Could you check a few things on this drawing? It's one solid part, dimensions in mm from its lowest x, y, z. Round coordinates to 2 decimals unless told otherwise and drop trailing zeros. Loops run counter-clockwise (first coordinate to the right, second up) from the corner with the lowest first, then second, coordinate; pieces in that order, holes last. Notation, with made-up numbers: (-37.75, -1.5) -> (-29.75, -1.5) arc R27 cw to (-29.75, 29.5) -> close; hole circle Ø8 at (8.25, 26.25). An arc over 180 degrees is marked (long way). Write each question's results on one line, items separated by ' | '.
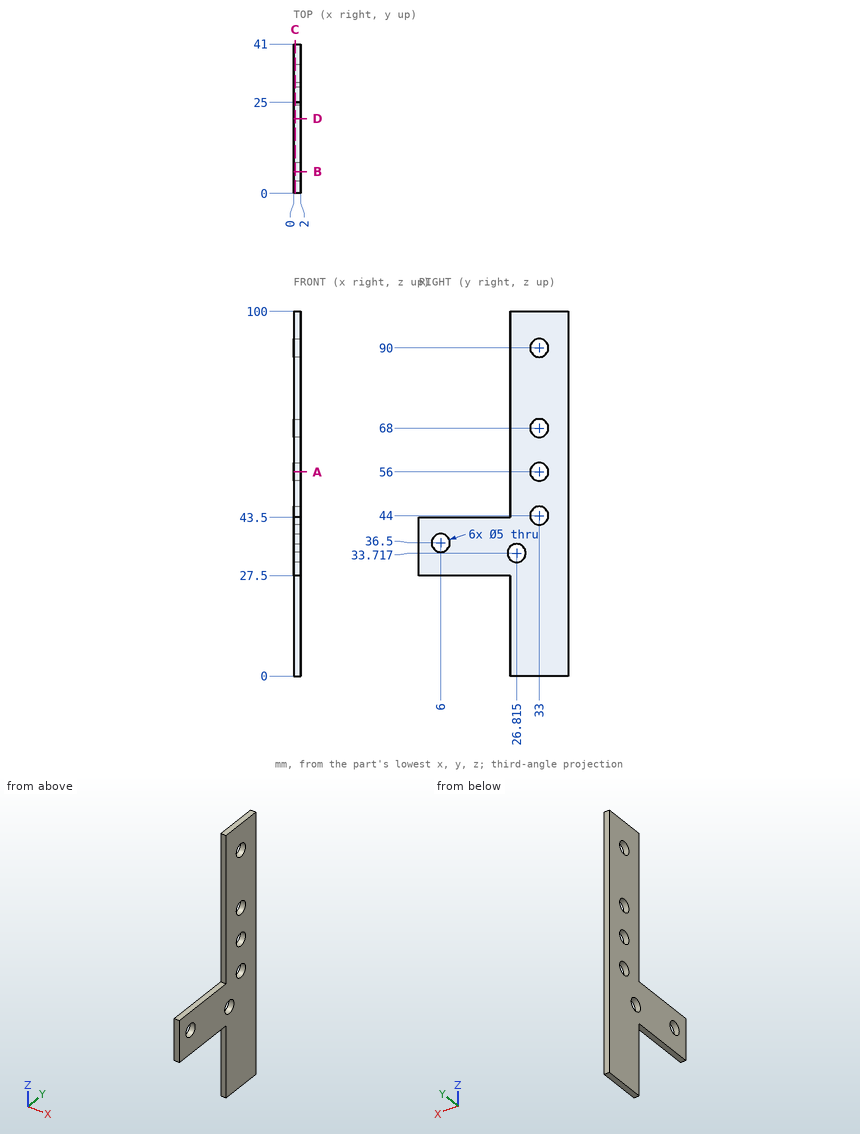
1) I'm going to push flat-ended pins straight in: pin 1 (4.5 mm diameter, centred on y = 26.81, z = 33.72, fed in from -X); pin 2 (0.6 mm diameter, centred on x = 1.5, z = 9, fed in from -Y). Where does each tip first touch, or does it pass through?
Model answer:
pin 1: passes through | pin 2: stops at y = 25
2) I want a section at B-B, the plane y = 6. Write out the boundary of the cut face in (x, z).
Model answer:
outline: (0, 27.5) -> (2, 27.5) -> (2, 34) -> (0, 34) -> close; (0, 39) -> (2, 39) -> (2, 43.5) -> (0, 43.5) -> close
3) I want a section at D-D, the plane y = 20.5. Write out the boundary of the cut face in (x, z), plus the area to 3 significant figures.
Model answer:
outline: (0, 27.5) -> (2, 27.5) -> (2, 43.5) -> (0, 43.5) -> close | area: 32.0 mm2
4) I need wall thicknesses on line 1 (Y direction, x = 1.45, z = 68); line 2 (Y direction, x = 0.7, z = 36.5); line 3 (Y direction, x = 1.4, z = 16). Which ranges of each line are inside material? Lowest first, please.
Model answer:
line 1: y = 25 to 30.5, 35.5 to 41 | line 2: y = 0 to 3.5, 8.5 to 41 | line 3: y = 25 to 41
5) I want a section at C-C, the plane x = 0.4. Write out the boundary of the cut face in (y, z) (1 decimal), plus the area to 3 significant figures.
Model answer:
outline: (0, 27.5) -> (25, 27.5) -> (25, 0) -> (41, 0) -> (41, 100) -> (25, 100) -> (25, 43.5) -> (0, 43.5) -> close; hole circle Ø5 at (6, 36.5); hole circle Ø5 at (26.8, 33.7); hole circle Ø5 at (33, 44); hole circle Ø5 at (33, 56); hole circle Ø5 at (33, 68); hole circle Ø5 at (33, 90) | area: 1,880 mm2
6) I want a section at A-A, the plane z = 56. Write out the boundary of the cut face in (x, y).
Model answer:
outline: (0, 25) -> (2, 25) -> (2, 30.5) -> (0, 30.5) -> close; (0, 35.5) -> (2, 35.5) -> (2, 41) -> (0, 41) -> close
